Design review of the part built by this model. Coordinates are the model's own, in mm. A direction names the side the tool comes from. Round coordinates to 2 decimals unless told otherwise and drop trailing zeros. Order: outer loops, then holes, each group sorted by start corner. A loop starts at its lowest first (then second) coordinate and runs counter-clockwise, first axis right, second up. Notation, with made-up numbers: (50.5, -21) - (61.5, -21) arc R7 cw to (61.5, -14) - close; hole circle Ø9 at (15, 70). An arc over 180 degrees is marked (long way). Use CSV: the item, a comma, the result in double quotes. Start each with the question number.
from build123d import *

# Parameters (mm, degrees)
SKETCH_1_R          = 17.55
EXTRUDE_1_DEPTH     = 2.1
EXTRUDE_START       = 2.1
SKETCH_2_R          = 14.8
SKETCH_2_R_2        = 6.1
EXTRUDE_2_DEPTH     = 3.3
CUT_EXTRUDE_1_REACH = 7.4
SKETCH_3_R          = 2.55
CHAMFER_1_SIZE      = 0.3


with BuildPart() as part:
    # 草图1 → 凸台-拉伸1 (new body)
    with BuildSketch(Plane.XY):
        Circle(SKETCH_1_R)
    extrude(amount=EXTRUDE_1_DEPTH)

    # 草图2 → 凸台-拉伸2 (add)
    with BuildSketch(Plane.XY.offset(EXTRUDE_START)):
        Circle(SKETCH_2_R)
        Circle(SKETCH_2_R_2, mode=Mode.SUBTRACT)
    extrude(amount=EXTRUDE_2_DEPTH)

    # 草图3 → 切除-拉伸1 (cut, up to next)
    with BuildSketch(Plane.XY, mode=Mode.PRIVATE) as cut_extrude_1_sk1:
        Circle(SKETCH_3_R)
    cut_extrude_1_tool1 = extrude(cut_extrude_1_sk1.sketch, amount=CUT_EXTRUDE_1_REACH, mode=Mode.PRIVATE) & part.part
    add(cut_extrude_1_tool1.solids().sort_by_distance((0, 0, 0))[0], mode=Mode.SUBTRACT)

    # 倒角1
    chamfer_1_edges = [part.edges().sort_by_distance(p)[0] for p in [
        (-2.55, 0, 2.1),
    ]]
    chamfer(chamfer_1_edges, length=CHAMFER_1_SIZE)


solid = part.part
Q1. Take a section at C-C (z = 2.55). State the section outline as (x, y) points.
Q2. For L1, parallel to Y at x = 0, z = 3.15; L2, parallel to Y at x = 0, z = 1.15; L3, parallel to Z at x = 3, y = 3.5, list the stretches that pass through material, from the lowest coordinate up. Write a range as [from, to].
Q3. Tool access review of faces 1 (the cylindrical face through (-6.094, 0.268, 3.727)), 2 (the cylindrical face through (-13.927, -10.679, 1.035)): name each direction out of +Z, -Z, +X, -X, +Y, -Y from which nothing blocks a thin tool from reaching the whole face with its end or side.
Q4. Take a section at A-A (x = 0). State the section outline as (y, z) points, plus the area to 3 significant figures.
Q5. Take a section at D-D (y = 11.5). State the section outline as (x, z) points, plus the area to 3 significant figures.
Q6. Clearance check with flat-ended pins moving along their axes: pin 1 (3 mm diameter, centred on x = -7, z = 4, fed in from +Y); pin 2 (6 mm diameter, centred on x = 0, y = 0, fed in from -Z); pin 3 (1 mm diameter, centred on y = -6, z = 0.5, fed in from -X); pin 4 (6 mm diameter, centred on x = -1.5, y = 1, fed in from +Z). State where each tip first meets the part, or that it passes through.
Q7. The part is to be moulded in two halves that separate along Y. For faces 3 (the cylindrical face through (1.18, -2.26, 0.89)), 4 (the flat face through (-9, -12, 2.1)), 5 (the flat face through (3, -1, 2.1)), 6 (the cylindrical face through (-3.208, -14.448, 3.727)), say which applies: +Y half, -Y half, draft (parallel to the pull), parting line (faces both ways), or undercut.
Findings below:
1,outline,"circle Ø29.6 at (0, 0); hole circle Ø12.2 at (0, 0)"
2,L1,"y = [-14.8, -6.1], [6.1, 14.8]"
2,L2,"y = [-17.55, -2.55], [2.55, 17.55]"
2,L3,"z = [0, 2.1]"
3,face 1,"+Z"
3,face 2,"+Z, -Z"
4,outline,"(-17.55, 0) - (-2.55, 0) - (-2.55, 1.8) - (-2.85, 2.1) - (-6.1, 2.1) - (-6.1, 5.4) - (-14.8, 5.4) - (-14.8, 2.1) - (-17.55, 2.1) - close; (2.55, 0) - (17.55, 0) - (17.55, 2.1) - (14.8, 2.1) - (14.8, 5.4) - (6.1, 5.4) - (6.1, 2.1) - (2.85, 2.1) - (2.55, 1.8) - close"
4,area,"120 mm^2"
5,outline,"(-13.26, 0) - (13.26, 0) - (13.26, 2.1) - (9.32, 2.1) - (9.32, 5.4) - (-9.32, 5.4) - (-9.32, 2.1) - (-13.26, 2.1) - close"
5,area,"117 mm^2"
6,pin 1,"stops at y = 13.74"
6,pin 2,"stops at z = 0"
6,pin 3,"stops at x = -16.67"
6,pin 4,"stops at z = 2.1"
7,face 3,"undercut"
7,face 4,"draft"
7,face 5,"undercut"
7,face 6,"parting line"
